from build123d import *

# Parameters (mm, degrees)
BOSS_EXTRUDE1_DEPTH = 470
SKETCH2_R           = 5
CUT_EXTRUDE1_DEPTH  = 506.766744656
BOSS_EXTRUDE2_DEPTH = 50
SKETCH4_W           = 70
SKETCH4_H           = 25
SKETCH4_W_2         = 10
CUT_EXTRUDE2_DEPTH  = 80
SKETCH6_W           = 17.656216206
SKETCH6_H           = 13.202094069
SKETCH6_R           = 4
BOSS_EXTRUDE3_DEPTH = 5


with BuildPart() as part:
    # Sketch1 → Boss-Extrude1 (new body)
    with BuildSketch(Plane.XY):
        Polygon((180, -50), (180, -60), (0, -60), (0, 0), (10, 0), (10, -50), align=None)
    extrude(amount=BOSS_EXTRUDE1_DEPTH)

    # Sketch2 → Cut-Extrude1 (cut, through all)
    with BuildSketch(Plane(origin=(0, -50, 0), x_dir=(1, 0, 0), z_dir=(0, 1, 0))):
        with Locations(Location((33.75, -235, 0), (0, 0, 270))):
            Circle(SKETCH2_R)
    extrude(amount=-CUT_EXTRUDE1_DEPTH, mode=Mode.SUBTRACT)

    # Sketch3 → Boss-Extrude2 (add)
    with BuildSketch(Plane(origin=(0, -50, 0), x_dir=(1, 0, 0), z_dir=(0, 1, 0))):
        Polygon((10, -460), (10, -470), (180, -470), (180, 0), (10, 0), (10, -10), (170, -10), (170, -460), align=None)
    extrude(amount=BOSS_EXTRUDE2_DEPTH)

    # Sketch4 → Cut-Extrude2 (cut, symmetric)
    with BuildSketch(Plane(origin=(0, -50, 0), x_dir=(1, 0, 0), z_dir=(0, 1, 0))):
        with Locations((135, -222.5)):
            Rectangle(SKETCH4_W, SKETCH4_H)
        with Locations((135, -247.5)):
            Rectangle(SKETCH4_W, SKETCH4_H)
        with Locations((175, -222.5)):
            Rectangle(SKETCH4_W_2, SKETCH4_H)
        with Locations((175, -247.5)):
            Rectangle(SKETCH4_W_2, SKETCH4_H)
    extrude(amount=CUT_EXTRUDE2_DEPTH, both=True, mode=Mode.SUBTRACT)

    # Sketch6 → Boss-Extrude3 (add)
    with BuildSketch(Plane.XY.offset(210)):
        with Locations((171.171891897, -66.601047034)):
            Rectangle(SKETCH6_W, SKETCH6_H)
        with Locations((170.838161539, -66.744917763)):
            Circle(SKETCH6_R, mode=Mode.SUBTRACT)
    boss_extrude3 = extrude(amount=-BOSS_EXTRUDE3_DEPTH)

    # Mirror1: Boss-Extrude3 across plane
    add(boss_extrude3.mirror(Plane.XY.offset(235)))


solid = part.part
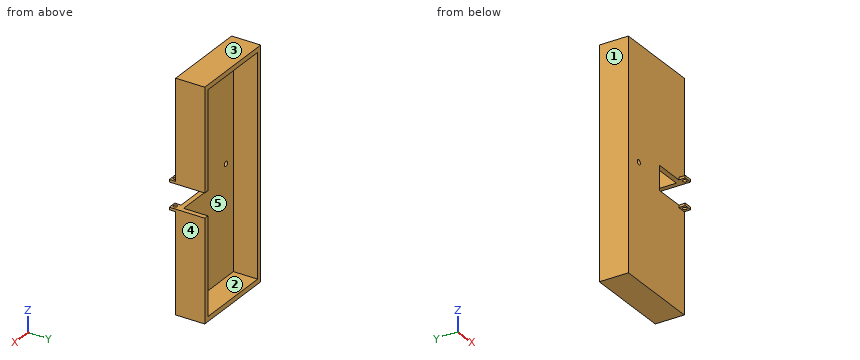
Can you work these out from the model? Positions are in its coordinate system, mm. Face numbers are marked on the shaded views. A direction names the side the tool comes from. Coordinates: 2 decimals unless noted, no trailing zeros. Write each loop counter-clockwise with the first axis right and the second up, starting at its lowest first coordinate (ties: lowest second). Pieces come first, ordered by that corner, then holes.
Q1. If we mould it in two halves opening along X, with no side actions, what happens to the marked faces 3, 4 and 5? For each: +X half, -X half, draft (parallel to the pull), parting line (faces both ways), or undercut.
Results found:
face 3: draft
face 4: +X half
face 5: undercut
Q2. For P1, Ø4, axis at y = -67, z = 262.5, coming from the -X side; P2, Ø11, axis at y = -53, z = 239, coming from the +X side; P3, Ø14.5, axis at x = 168.5, y = -67.5, coming from the +Z side, each with a flat end and sliding along its axis, tell me the tip position at first contact or that it passes through.
Results found:
P1: stops at x = 162.34
P2: stops at x = 100
P3: stops at z = 265
Q3. Which directions (+Z, -Z, +X, -X, +Y, -Y) give clear straight access to the entire face, cutting with the end or side of a thin tool? Please do the marked faces 1 and 2.
Results found:
face 1: +Z, -Z, -X, +Y, -Y
face 2: +Y
Q4. Imagine slicing it at B-B, the plane z = 235. List the corners of the cut face in (x, y) for me, plus the area to 3 significant figures.
Results found:
outline: (0, -60) - (28.75, -60) - (28.75, -50) - (10, -50) - (10, 0) - (0, 0) - close; (38.75, -60) - (100, -60) - (100, -50) - (38.75, -50) - close
area: 1,400 mm2
Q5. Imagine slicing it at C-C, the plane y = -35.5. List the corners of the cut face in (x, z) for me, plus the area to 3 significant figures.
Results found:
outline: (0, 0) - (180, 0) - (180, 210) - (170, 210) - (170, 10) - (10, 10) - (10, 460) - (170, 460) - (170, 260) - (180, 260) - (180, 470) - (0, 470) - close
area: 12,100 mm2
Q6. Imagine slicing it at D-D, the plane z = 179. List the corners of the cut face in (x, y) for me, plus the area to 3 significant figures.
Results found:
outline: (0, -60) - (180, -60) - (180, 0) - (170, 0) - (170, -50) - (10, -50) - (10, 0) - (0, 0) - close
area: 2,800 mm2
Q7. Imagine slicing it at A-A, the plane x = 135. List the corners of the cut face in (y, z) for me.
Results found:
outline: (-60, 0) - (0, 0) - (0, 10) - (-50, 10) - (-50, 210) - (-60, 210) - close; (-60, 260) - (-50, 260) - (-50, 460) - (0, 460) - (0, 470) - (-60, 470) - close
Q8. Please list where these lines run through material, in increasing order: L1, parallel to X at y = -52, z = 235; L2, parallel to X at y = -29, z = 399; L3, parallel to Z at x = 63, y = -24.5.
Results found:
L1: x = 0 to 28.75, 38.75 to 100
L2: x = 0 to 10, 170 to 180
L3: z = 0 to 10, 460 to 470
